Read the model definition and answer for the solid it produces. Units are mm, in the model's axes. Face numbers are marked on the shaded views. Give positions to 0.01 mm unless a question says otherwise; leave off trailing zeros. Write each loop counter-clockwise with the first axis right and the second up, starting at its lowest first coordinate (ties: lowest second). Pieces come first, ordered by that corner, then holes. Notation, with made-up numbers: (-1.75, 44.25) -> (15.25, 44.25) arc R8 cw to (15.25, 49.25) -> close; hole circle Ø3 at (-31.75, 51). An arc over 180 degrees is marked (long way). Answer as CSV lines item,"result". Start each with the question number.
1. Given pin 1 (7.5 mm diameter, centred on x = -130.5, y = 37, fed in from +Z), flat-ended and moving along its own axis, determine where the tip first touches the part or whether it passes through.
2. The part is cut by section C-C, the plane y = -10.5. Determine the outline of the cut face in (x, z), and give its area (3 significant figures).
3. The part is cut by section B-B, the plane x = -50. Determine the outline of the cut face in (y, z).
4. Find the intervals of material crossed by line 1 (Y direction, x = -144, z = 1.4); line 2 (X direction, y = 32, z = 2.3); line 3 (Z direction, x = -36, y = -3), in increasing order.
5. The part is cut by section A-A, the plane z = 2.3. Determine the outline of the cut face in (x, y), and give its area (3 significant figures).
6. For a pull along X with two mould halves and no side action, classify the marked faces 1 and 2 as pulls with the +X half, pulls with the -X half, needs draft (parallel to the pull), parting line crosses it, or undercut.
from build123d import *

# Parameters (mm, degrees)
CROQUIS1_W              = 143
CROQUIS1_H              = 82
SALIENTE_EXTRUIR1_DEPTH = 1
CROQUIS2_W              = 143
CROQUIS2_H              = 82
CROQUIS2_W_2            = 141
CROQUIS2_H_2            = 80
CROQUIS2_W_3            = 139
CROQUIS2_H_3            = 78
CROQUIS2_W_4            = 136
CROQUIS2_H_4            = 25.104148451
CROQUIS2_H_5            = 49.895851549
SALIENTE_EXTRUIR2_DEPTH = 2


with BuildPart() as part:
    # Croquis1 → Saliente-Extruir1 (new body)
    with BuildSketch(Plane.XY):
        with Locations((-99.522825922, 14.293939394)):
            Rectangle(CROQUIS1_W, CROQUIS1_H)
    extrude(amount=SALIENTE_EXTRUIR1_DEPTH)

    # Croquis2 → Saliente-Extruir2 (add)
    with BuildSketch(Plane.XY.offset(1)):
        with Locations((-99.522825922, 14.293939394)):
            Rectangle(CROQUIS2_W, CROQUIS2_H)
        with Locations((-99.522825922, 14.293939394)):
            Rectangle(CROQUIS2_W_2, CROQUIS2_H_2, mode=Mode.SUBTRACT)
        with Locations((-99.522825922, 14.293939394)):
            Rectangle(CROQUIS2_W_3, CROQUIS2_H_3)
        with Locations((-100.022825922, 39.741865169)):
            Rectangle(CROQUIS2_W_4, CROQUIS2_H_4, mode=Mode.SUBTRACT)
        with Locations((-100.022825922, 1.241865169)):
            Rectangle(CROQUIS2_W_4, CROQUIS2_H_5, mode=Mode.SUBTRACT)
    extrude(amount=SALIENTE_EXTRUIR2_DEPTH)


solid = part.part
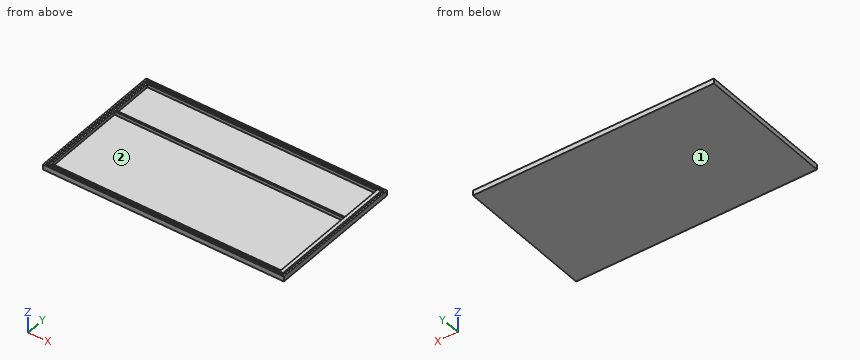
Results found:
1,pin 1,"stops at z = 1"
2,outline,"(-171.02, 0) -> (-28.02, 0) -> (-28.02, 3) -> (-29.02, 3) -> (-29.02, 1) -> (-30.02, 1) -> (-30.02, 3) -> (-32.02, 3) -> (-32.02, 1) -> (-168.02, 1) -> (-168.02, 3) -> (-169.02, 3) -> (-169.02, 1) -> (-170.02, 1) -> (-170.02, 3) -> (-171.02, 3) -> close"
2,area,"153 mm²"
3,outline,"(-26.71, 0) -> (55.29, 0) -> (55.29, 3) -> (54.29, 3) -> (54.29, 1) -> (53.29, 1) -> (53.29, 3) -> (52.29, 3) -> (52.29, 1) -> (27.19, 1) -> (27.19, 3) -> (26.19, 3) -> (26.19, 1) -> (-23.71, 1) -> (-23.71, 3) -> (-24.71, 3) -> (-24.71, 1) -> (-25.71, 1) -> (-25.71, 3) -> (-26.71, 3) -> close"
4,line 1,"y = -26.71 to -25.71, -24.71 to -23.71, 26.19 to 27.19, 52.29 to 53.29, 54.29 to 55.29"
4,line 2,"x = -171.02 to -170.02, -169.02 to -168.02, -32.02 to -30.02, -29.02 to -28.02"
4,line 3,"z = 0 to 1"
5,outline,"(-171.02, -26.71) -> (-28.02, -26.71) -> (-28.02, 55.29) -> (-171.02, 55.29) -> close; (-169.02, -24.71) -> (-30.02, -24.71) -> (-30.02, 53.29) -> (-169.02, 53.29) -> close; hole (-170.02, -25.71) -> (-29.02, -25.71) -> (-29.02, 54.29) -> (-170.02, 54.29) -> close; hole (-168.02, -23.71) -> (-32.02, -23.71) -> (-32.02, 26.19) -> (-168.02, 26.19) -> close; hole (-168.02, 27.19) -> (-32.02, 27.19) -> (-32.02, 52.29) -> (-168.02, 52.29) -> close"
5,area,"1,090 mm²"
6,face 1,"needs draft"
6,face 2,"undercut"
